Work out the finished part from the listing and answer in its coordinate system (mm). Face numbers are marked on the shaded views. A direction names the side the tool comes from. Round coordinates to 2 decimals unless told otherwise and drop trailing zeros. Loops run counter-clockwise (first coordinate to the right, second up) from the corner with the lowest first, then second, coordinate; pieces in that order, holes last. Notation, with made-up numbers: (75, 67) -> (107, 67) arc R20 cw to (107, 91) -> close; hole circle Ø10 at (31, 45). An arc over 180 degrees is marked (long way). Use CSV: the item, a comma, the result in double quotes. Start each with the question number.
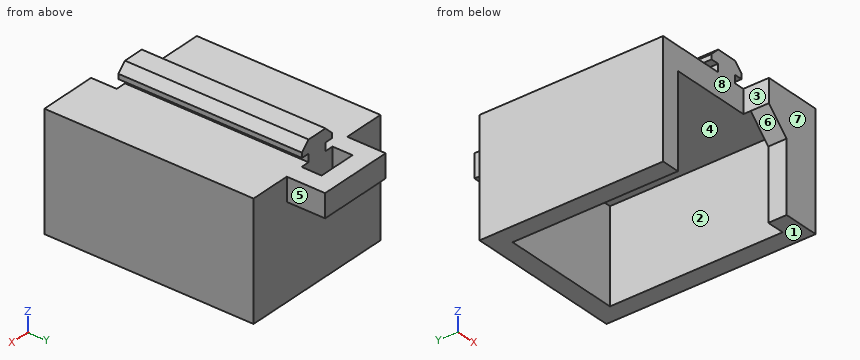
from build123d import *

# Parameters (mm, degrees)
BOSS_EXTRUDE1_DEPTH = 25.2
BOSS_EXTRUDE2_DEPTH = 6.35
BOSS_EXTRUDE3_START = 2
BOSS_EXTRUDE3_DEPTH = 5
SKETCH4_W           = 6
SKETCH4_H           = 2
BOSS_EXTRUDE4_DEPTH = 6.35
BOSS_EXTRUDE5_DEPTH = 50.228


with BuildPart() as part:
    # Sketch1 → Boss-Extrude1 (new body)
    with BuildSketch(Plane.XY):
        Polygon((-16.5, -29.728), (-16.5, 15.5), (16.5, 15.5), (16.5, -28.399762486), (16.5, -31.728), (11.67, -31.728), (11.67, -36.728), (21.5, -36.728), (21.5, 20.5), (-21.5, 20.5), (-21.5, -29.728), align=None)
    extrude(amount=-BOSS_EXTRUDE1_DEPTH)

    # Sketch2 → Boss-Extrude2 (add)
    with BuildSketch(Plane.XY):
        Polygon((-21.5, 20.5), (21.5, 20.5), (21.5, -29.728), (21.5, -36.728), (11.67, -36.728), (11.67, -29.728), (-21.5, -29.728), align=None)
    extrude(amount=BOSS_EXTRUDE2_DEPTH)

    # Sketch3 → Boss-Extrude3 (add)
    with BuildSketch(Plane.XZ.offset(29.728).offset(BOSS_EXTRUDE3_START)):
        Polygon((11.67, 6.35), (5.67, 6.35), (5.67, 0), (11.67, -6), align=None)
    extrude(amount=BOSS_EXTRUDE3_DEPTH)

    # Sketch4 → Boss-Extrude4 (add)
    with BuildSketch(Plane.XY.offset(6.35)):
        Polygon((-10.25, 20.5), (-5.25, 20.5), (-5.25, 26), (5.25, 26), (5.25, 20.5), (10.25, 20.5), (10.25, 31), (-10.25, 31), align=None)
        with Locations((8.67, -30.728)):
            Rectangle(SKETCH4_W, SKETCH4_H)
    extrude(amount=-BOSS_EXTRUDE4_DEPTH)

    # Sketch5 → Boss-Extrude5 (add)
    with BuildSketch(Plane(origin=(0, 20.5, 0), x_dir=(1, 0, 0), z_dir=(0, 1, 0))):
        Polygon((-2.86, -6.35), (-2.86, -8.51), (-5.08, -8.51), (-5.08, -9.85), (-2.86, -12.07), (2.86, -12.07), (5.08, -9.85), (5.08, -8.51), (2.86, -8.51), (2.86, -6.35), align=None)
    extrude(amount=-BOSS_EXTRUDE5_DEPTH)


solid = part.part
Q1. Section D-D, the plane x = -6 is taken. Write down the section's boundary in (y, z).
Q2. Straight lines are drawn through the part: line 1 (X direction, y = -25, z = -3); line 2 (Y direction, x = 13, z = -18); line 3 (Z direction, x = -17.5, y = -8.5). For each, find the intervals that lie inside material, in ascending order. Write a range as from..to.
Q3. Section C-C, the plane x = 1.5 is taken. Write down the section's boundary in (y, z), and give its area (3 significant figures).
Q4. Section B-B, the plane z = 1 is taken. Write down the section's boundary in (x, y), and give its area (3 significant figures).
Q5. Which of the six approach directions +Z, -Z, +X, -X, +Y, -Y give full straight-line access (tool end or side, diameter ignored) to the marked faces 4, 5, 6, 7 and 8?
Q6. Each of these flat-tipped pins is pushed along its axis until it touches: pin 1 (2.5 mm diameter, centred on y = -34, z = -19.5, fed in from -X); pin 2 (7 mm diameter, centred on y = 26.5, z = 3.5, fed in from -X); pin 3 (5 mm diameter, centred on x = 1.5, z = 3.5, fed in from -Y). Where does it stop, or does it pass through?
Q7. Section A-A, the plane y = 25 is taken. Write down the section's boundary in (x, z).
Q8. For a pull along X with two mould halves and no side action, classify the marked faces 1, 2 and 3 as pulls with the +X half, pulls with the -X half, needs draft (parallel to the pull), parting line crosses it, or undercut.
Report:
1,outline,"(-29.73, 0) -> (15.5, 0) -> (15.5, -25.2) -> (20.5, -25.2) -> (20.5, 0) -> (31, 0) -> (31, 6.35) -> (-29.73, 6.35) -> close"
2,line 1,"x = -21.5..-16.5, 16.5..21.5"
2,line 2,"y = -36.73..-31.73, 15.5..20.5"
2,line 3,"z = -25.2..6.35"
3,outline,"(-29.73, 0) -> (15.5, 0) -> (15.5, -25.2) -> (20.5, -25.2) -> (20.5, 12.07) -> (-29.73, 12.07) -> close; (26, 0) -> (31, 0) -> (31, 6.35) -> (26, 6.35) -> close"
3,area,"764 mm²"
4,outline,"(-21.5, -29.73) -> (5.67, -29.73) -> (5.67, -36.73) -> (21.5, -36.73) -> (21.5, 20.5) -> (10.25, 20.5) -> (10.25, 31) -> (-10.25, 31) -> (-10.25, 20.5) -> (-21.5, 20.5) -> close; hole (-5.25, 20.5) -> (5.25, 20.5) -> (5.25, 26) -> (-5.25, 26) -> close"
4,area,"2,430 mm²"
5,face 4,"-Z"
5,face 5,"+Z, -Z, +X, +Y"
5,face 6,"-Z, -X, -Y"
5,face 7,"+Z, -Z, +X, -X, -Y"
5,face 8,"+Z, -Z, -X, -Y"
6,pin 1,"stops at x = 11.67"
6,pin 2,"stops at x = -10.25"
6,pin 3,"stops at y = -29.73"
7,outline,"(-10.25, 0) -> (-5.25, 0) -> (-5.25, 6.35) -> (-10.25, 6.35) -> close; (5.25, 0) -> (10.25, 0) -> (10.25, 6.35) -> (5.25, 6.35) -> close"
8,face 1,"needs draft"
8,face 2,"undercut"
8,face 3,"pulls with the -X half"
